Verification items for the finished model (mm, model axes). A direction names the side the tool comes from. Give positions to 0.01 mm unless a question says otherwise; leave off trailing zeros. Loops run counter-clockwise (first coordinate to the right, second up) from the corner with the lowest first, then second, coordinate; pieces in that order, holes last. Notation, with made-up numbers: M 20.5,-29.5 L 58.5,-29.5 A29 ccw 58.5,-6.5 Z; hole C 32.5,-6 d3. An arc over 180 degrees is marked long. Write each question's results on one line, items separated by ' | '. Start each with the question number.
Autodesk Inventor part; units mm, degrees
ref_plane "YZ Plane" through (0, 0, 0) normal (1, 0, 0) x (0, 1, 0)
ref_plane "XZ Plane" through (0, 0, 0) normal (0, 1, 0) x (-1, 0, 0)
ref_plane "XY Plane" through (0, 0, 0) normal (0, 0, 1) x (1, 0, 0)
sketch "Sketch1" plane through (0, 0, 0) normal (0, 1, 0) x (-1, 0, 0)
  circle A0 centre (0, 0) radius 3
  dimension "d0" = 6
extrude "Extrusion1" add sketch "Sketch1" along normal blind 6
sketch "Sketch2" plane through (0, 0, 0) normal (0, -1, 0) x (1, 0, 0)
  circle A0 centre (0, 0) radius 0.75
  circle A1 centre (0, 0) radius 3
  dimension "d3" = 1.5
extrude "Extrusion2" cut sketch "Sketch2" against normal blind 1
loft "Loft1" add section 1 edges at (-0.75, 0, 0) section 2 edges at (3, 1, 0)
thread "Thread1"
sketch "Sketch3" plane through (0, 6, 0) normal (0, 1, 0) x (1, 0, 0)
  line L0 (0, 0) -> (0, 1.5)
  line L1 (0, 1.5) -> (1.299, 0.75)
  line L2 (1.299, 0.75) -> (1.299, -0.75)
  line L3 (1.299, -0.75) -> (0, -1.5)
  line L4 (0, -1.5) -> (-1.299, -0.75)
  line L5 (-1.299, -0.75) -> (-1.299, 0.75)
  line L6 (-1.299, 0.75) -> (0, 1.5)
  dimension "d12" = 1.5
extrude "Extrusion3" cut sketch "Sketch3" against normal blind 2
properties part number "M6x6_DIN914" material "Steel, Mild"
1. Release check for a two-part mould opening along Z. For faces 1 (the face through (3, 3, 0)), 2 (the face through (-0.64, 5.01, 1.13)), 3 (the face through (0, 0, 0)) record: released by +Z, released by -Z, zero draft, split by the parting line, or undercut.
2. Set-up check for faces 4 (the face through (-0.193, 0.063, 0.87)), 5 (the face through (0, 4, 0)): record each of +Z, -Z, +X, -X, +Y, -Y from which the full face is reachable in a straight line by a thin tool's end or side.
3. Depth check by flat-ended pin: pin 1 Ø1.3 at (x, z) = (-0.5, 0) entering from +Y; pin 2 Ø1 at (x, y) = (-1.5, 3.5) entering from +Z; pin 3 Ø2 at (y, z) = (4.5, 1.5) entering from +X. Enter the tip coordinate at first touch or a pass-through.
4. Section check B-B, the plane y = 1.75. Record the boundary of the cut face in (x, z).
5. Section check A-A, the plane y = 4.5. Record the boundary of the cut face in (x, z), plus the area to 3 significant figures.
6. Thickness scan on probe 1 along X at (y, z) = (5.75, -0.25); probe 2 along Z at (x, y) = (2.25, 3); probe 3 along Y at (x, z) = (-1.25, -1.25). Record the ranges inside material, lowest first.
Filled sheet:
1) face 1: split by the parting line | face 2: undercut | face 3: zero draft
2) face 4: -Y | face 5: +Y
3) pin 1: y = 4 | pin 2: z = 2.83 | pin 3: x = 2.96
4) outline: C 0,0 d6
5) outline: C 0,0 d6; hole M -1.3,-0.75 L 0,-1.5 L 1.3,-0.75 L 1.3,0.75 L 0,1.5 L -1.3,0.75 Z | area: 22.4 mm2
6) probe 1: -2.99 to -1.3, 1.3 to 2.99 | probe 2: -1.98 to 1.98 | probe 3: 0.45 to 6
